Source: CAD feature listing. Evaluate the final solid. Frame: model axes, mm. A direction names the side the tool comes from. Give positions to 0.01 mm unless a question says otherwise; leave off trailing zeros. Order: outer loops, then holes, each group sorted by start corner. A loop starts at its lowest first (then second) coordinate and runs counter-clockwise, first axis right, second up.
from build123d import *

# Parameters (mm, degrees)
SKETCH_1_R      = 1.65
SKETCH_1_R_2    = 1.620295374
EXTRUDE_1_DEPTH = 3
FILLET_1_R      = 5


with BuildPart() as part:
    # 草图1 → 凸台-拉伸1 (new body)
    with BuildSketch(Plane.XY):
        Polygon((-4.38586222, 10.641032467), (27.611336651, 34.638936735), (27.610889092, -35.358299417), (7.610889171, -35.358299417), (7.614139416, -5.358966306), (-16.385858742, -23.358968761), (-28.385860379, -7.358969988), align=None)
        with Locations((17.724788113, 14.641700583)):
            Circle(SKETCH_1_R, mode=Mode.SUBTRACT)
        with Locations((17.610953032, -5.358299417)):
            Circle(SKETCH_1_R_2, mode=Mode.SUBTRACT)
        with Locations((17.610953032, -25.358299417)):
            Circle(SKETCH_1_R, mode=Mode.SUBTRACT)
        with Locations((-6.385860788, -3.358967738)):
            Circle(SKETCH_1_R, mode=Mode.SUBTRACT)
        with Locations((-14.385860174, -9.358968556)):
            Circle(SKETCH_1_R, mode=Mode.SUBTRACT)
    extrude(amount=EXTRUDE_1_DEPTH)

    # 圆角1
    fillet_1_edges = [part.edges().sort_by_distance(p)[0] for p in [
        (27.611336651, 34.638936735, 1.5),
        (7.614139416, -5.358966306, 1.5),
    ]]
    fillet(fillet_1_edges, radius=FILLET_1_R)


solid = part.part
1) Section query C-C on x = -9. Output: boundary loops of the cut face in (y, z).
Checks:
outline: (-17.82, 0) - (7.18, 0) - (7.18, 3) - (-17.82, 3) - close
2) Reachability of faces 4 (the face through (-8.274, -17.275, 1.479)), 5 (the face through (18, -35.358, 1)) from +Z, -Z, +X, -X, +Y, -Y: full face, straight path, thin tool, end or side. Return the list, or none.
Checks:
face 4: +Z, -Z, -Y
face 5: +Z, -Z, +X, -X, -Y
3) Section query B-B on z = 2.3. Output: boundary loops of the cut face in (x, y).
Checks:
outline: (-28.39, -7.36) - (-16.39, -23.36) - (-0.39, -11.36) arc R5 cw to (7.61, -15.36) - (7.61, -35.36) - (27.61, -35.36) - (27.61, 24.64) arc R5 ccw to (19.61, 28.64) - close; hole circle Ø3.3 at (-14.39, -9.36); hole circle Ø3.3 at (-6.39, -3.36); hole circle Ø3.3 at (17.61, -25.36); hole circle Ø3.24 at (17.61, -5.36); hole circle Ø3.3 at (17.72, 14.64)
4) First-contact query: pin 1 Ø1.5 at (x, z) = (-14, 1.5) entering from -Y; pin 2 Ø1.5 at (y, z) = (-25.5, 1) entering from -X. Flat tips, straight axial feed; report the tip coordinate or a pass-through.
Checks:
pin 1: stops at y = -22.13
pin 2: stops at x = 7.61
5) Ray query, L1, parallel to Y at x = 16.5, z = 0.3; L2, parallel to X at y = -19.5, z = 1.55; L3, parallel to Y at x = 23, z = 2.1. Return the intervals inside material, ascending.
Checks:
L1: y = -35.36 to -26.58, -24.14 to -6.54, -4.18 to 13.54, 15.75 to 26.31
L2: x = -19.28 to -11.24, 7.61 to 27.61
L3: y = -35.36 to 29.62
6) Section query D-D on y = -29.5. Output: boundary loops of the cut face in (x, z).
Checks:
outline: (7.61, 0) - (27.61, 0) - (27.61, 3) - (7.61, 3) - close
7) Pull-direction query (X, two-part tool) for faces 1 (the face through (6, -2, 3)), 2 (the face through (17.25, -26.97, 1.48)), 3 (the face through (-22.302, -15.471, 1.479)); classes: +X half, -X half, draft (parallel to the pull), parting line (faces both ways), or undercut.
Checks:
face 1: draft
face 2: undercut
face 3: -X half
8) Section query A-A on y = -18.5. Output: boundary loops of the cut face in (x, z), and give its area (3 significant figures).
Checks:
outline: (-20.03, 0) - (-9.91, 0) - (-9.91, 3) - (-20.03, 3) - close; (7.61, 0) - (27.61, 0) - (27.61, 3) - (7.61, 3) - close
area: 90.4 mm2
